Geometry: final body of the model. Coordinates: model frame, mm. A direction names the side the tool comes from. Round coordinates to 2 decimals unless told otherwise and drop trailing zeros. Order: outer loops, then holes, each group sorted by start corner. A loop starts at its lowest first (then second) coordinate and runs counter-clockwise, first axis right, second up. Notation, with made-up numbers: M 60.25,-19.75 L 109.25,-19.75 A19 ccw 109.25,17.25 Z; hole C -13.75,68.5 d1. An arc over 180 degrees is marked long. Return JSON: item names as keys, results as strings. Group by question number.
Q1. Access query for faces 5 (the face through (0.578, -9.748, 15.141)), 6 (the face through (-9, -2.5, 9)), 7 (the face through (9, -2.5, 9)). Directions: +Z, -Z, +X, -X, +Y, -Y. A direction counts if a zero-diameter tool reaches every point of the face in a straight line with its end or side. Return the directions, or none.
Q2. Cut plane B-B on x = -0.5. Output: boundary loops of the cut face in (y, z).
Q3. Contact query for flat-ended pins moving along their axis: pin 1 (3 mm diameter, centred on x = 9, z = 10.5, fed in from +Y); pin 2 (3 mm diameter, centred on x = -8.5, z = 10.5, fed in from -Y); pin 3 (1.3 mm diameter, centred on x = 9.5, z = 5.5, fed in from -Y). Output: stop coordinate, or through.
Q4. Mould query, pull axis Y, two halves, no side actions, for faces 1 (the face through (0, 1, 18.1)), 2 (the face through (0, -11, 9)), 3 (the face through (-7, 0, 9)), 4 (the face through (0, 11, 9)). Classes: released by +Y, released by -Y, zero draft, split by the parting line, or undercut.
Q5. Ray query, probe 1 along Y at (x, z) = (8.75, 4.5); probe 2 along X at (y, z) = (1.75, 3); probe 3 along Y at (x, z) = (-9.5, 14). Return the intervals inside material, ascending.
Q6. Cut plane A-A on z = 5. Output: boundary loops of the cut face in (x, y).
Q7. Cut plane C-C on y = -9.25. Count the separate pieces of the cut face and the enclosed holes in it, and give its area (3 significant figures).
```python
from build123d import *

# Parameters (mm, degrees)
ESQUISSE1_R             = 11
BOSS_EXTRU_1_DEPTH      = 18.1
ENL_V_MAT_EXTRU_2_DEPTH = 24.866503724
ENL_V_START             = -4
ENL_V_MAT_EXTRU_3_DEPTH = 4
CONG_1_R                = 0.5
ESQUISSE6_R             = 0.5
BOSS_EXTRU_2_DEPTH      = 4


with BuildPart() as part:
    # Esquisse1 → Boss.-Extru.1 (new body)
    with BuildSketch(Plane.XY):
        with Locations(Location((0, 0, 0), (0, 0, 180))):
            Circle(ESQUISSE1_R)
    extrude(amount=BOSS_EXTRU_1_DEPTH)

    # Esquisse4 → Enlèv. mat.-Extru.2 (cut, through all)
    with BuildSketch(Plane.XY.offset(18.1)):
        with BuildLine():
            Line((10.712142643, 2.5), (7, 2.5))
            Line((7, 2.5), (7, -2.5))
            Line((7, -2.5), (10.712142643, -2.5))
            ThreePointArc((10.712142643, -2.5), (11, 0), (10.712142643, 2.5))
        make_face()
        with BuildLine():
            Line((-10.712142643, -2.5), (-7, -2.5))
            Line((-7, -2.5), (-7, 2.5))
            Line((-7, 2.5), (-10.712142643, 2.5))
            ThreePointArc((-10.712142643, 2.5), (-11, 0), (-10.712142643, -2.5))
        make_face()
    extrude(amount=-ENL_V_MAT_EXTRU_2_DEPTH, mode=Mode.SUBTRACT)

    # Esquisse5 → Enlèv. mat.-Extru.3 (cut)
    with BuildSketch(Plane.XY.offset(18.1).offset(ENL_V_START)):
        with BuildLine():
            Line((-7.549834435, -8), (7.549834435, -8))
            ThreePointArc((7.549834435, -8), (0, -11), (-7.549834435, -8))
        make_face()
    extrude(amount=ENL_V_MAT_EXTRU_3_DEPTH, mode=Mode.SUBTRACT)

    # Congé1
    cong_1_edges = [part.edges().sort_by_distance(p)[0] for p in [
        (10.712142643, 2.5, 9.05),
        (10.712142643, -2.5, 9.05),
        (7, -2.5, 9.05),
        (7, 2.5, 9.05),
        (-10.712142643, -2.5, 9.05),
        (-10.712142643, 2.5, 9.05),
        (-7, 2.5, 9.05),
        (-7, -2.5, 9.05),
    ]]
    fillet(cong_1_edges, radius=CONG_1_R)

    # Esquisse6 → Boss.-Extru.2 (add)
    with BuildSketch(Plane(origin=(0, -11.05, 11.05), x_dir=(-1, 0, 0), z_dir=(0, -0.7071067811865464, 0.7071067811865488))):
        with Locations(Location((0.6, -4.313351365, 0), (0, 0, 180))):
            Circle(ESQUISSE6_R)
        with Locations(Location((1.8, -4.313351365, 0), (0, 0, 180))):
            Circle(ESQUISSE6_R)
        with Locations(Location((3, -4.313351365, 0), (0, 0, 180))):
            Circle(ESQUISSE6_R)
        with Locations(Location((-3, -4.313351365, 0), (0, 0, 270))):
            Circle(ESQUISSE6_R)
        with Locations(Location((-1.8, -4.313351365, 0), (0, 0, 270))):
            Circle(ESQUISSE6_R)
        with Locations(Location((-0.6, -4.313351365, 0), (0, 0, 270))):
            Circle(ESQUISSE6_R)
    extrude(amount=BOSS_EXTRU_2_DEPTH)


solid = part.part
```
Result sheet:
{
 "1": {"face 5": "none", "face 6": "+Z, -Z, -X", "face 7": "+Z, -Z, +X"},
 "2": {"outline": "M -11.17,16.58 L -8.69,14.1 L -10.99,14.1 L -10.99,0 L 10.99,0 L 10.99,18.1 L -8,18.1 L -8,14.79 L -10.48,17.27 Z"},
 "3": {"pin 1": "stops at y = 8.05", "pin 2": "stops at y = -8.49", "pin 3": "stops at y = -6.53"},
 "4": {"face 1": "zero draft", "face 2": "released by -Y", "face 3": "undercut", "face 4": "released by +Y"},
 "5": {"probe 1": "y = -6.67 to -2.5, 2.5 to 6.67", "probe 2": "x = -7 to 7", "probe 3": "y = -5.55 to -2.5, 2.5 to 5.55"},
 "6": {"outline": "M -10.54,-3.14 A11 ccw 10.54,-3.14 A0.5 ccw 10.06,-2.5 L 7.5,-2.5 A0.5 cw 7,-2 L 7,2 A0.5 cw 7.5,2.5 L 10.06,2.5 A0.5 ccw 10.54,3.14 A11 ccw -10.54,3.14 A0.5 ccw -10.06,2.5 L -7.5,2.5 A0.5 cw -7,2 L -7,-2 A0.5 cw -7.5,-2.5 L -10.06,-2.5 A0.5 ccw Z"},
 "7": {"separate pieces": "7", "enclosed holes": "0", "area": "175 mm²"}
}
